The model under review builds one solid part; all positions refer to its coordinate system, in mm. A direction names the side the tool comes from. Give positions to 0.01 mm unless a question says otherwise; leave off trailing zeros. Write each loop counter-clockwise with the first axis right and the second up, starting at its lowest first coordinate (ties: lowest second). Pieces come first, ordered by that corner, then holes. Notation, with made-up numbers: M 68,-38 L 98,-38 A22 cw 98,-18 Z; hole C 12,79 d2. An arc over 180 degrees is marked long. Write item = value, one per line. Start each with the question number.
```python
from build123d import *

# Parameters (mm, degrees)
SKETCH1_W           = 10
SKETCH1_H           = 50
BOSS_EXTRUDE1_DEPTH = 2
SKETCH2_R           = 3
CUT_EXTRUDE1_DEPTH  = 2
SKETCH3_R           = 3
BOSS_EXTRUDE2_DEPTH = 20


with BuildPart() as part:
    # Sketch1 → Boss-Extrude1 (new body)
    with BuildSketch(Plane(origin=(0, 0, 0), x_dir=(0, 0, -1), z_dir=(1, 0, 0))):
        Rectangle(SKETCH1_W, SKETCH1_H)
    extrude(amount=BOSS_EXTRUDE1_DEPTH)

    # Sketch2 → Cut-Extrude1 (cut)
    with BuildSketch(Plane(origin=(2, 0, 0), x_dir=(0, 0, -1), z_dir=(1, 0, 0))):
        with Locations((0, 20)):
            Circle(SKETCH2_R)
    extrude(amount=-CUT_EXTRUDE1_DEPTH, mode=Mode.SUBTRACT)

    # Sketch3 → Boss-Extrude2 (add)
    with BuildSketch(Plane(origin=(2, 0, 0), x_dir=(0, 0, -1), z_dir=(1, 0, 0))):
        with Locations((0, -20)):
            Circle(SKETCH3_R)
    extrude(amount=BOSS_EXTRUDE2_DEPTH)


solid = part.part
```
Item 1: For faces 1 (the cylindrical face through (11.86, -22.93, 0.65)), 2 (the flat face through (22, -20, 0)), list the 3-axis set-ups (+Z, -Z, +X, -X, +Y, -Y) from which the entire face can be reached by the end or side of a thin tool; tool diameter is ignored.
Item 2: Clearance check with flat-ended pins moving along their axes: P1, Ø3.5, axis at y = 20, z = 0, coming from the -X side; P2, Ø5, axis at x = 10.5, z = -3.5, coming from the -Y side; P3, Ø6, axis at x = 14, y = -19.5, coming from the +Z side. State where each tip first meets the part, or that it passes through.
Item 3: We need section B-B, the plane y = 20. Write out the cut boundary in (x, z), and give its area (3 significant figures).
Item 4: We need section D-D, the plane x = 10.5. Write out the cut boundary in (y, z).
Item 5: We need section A-A, the plane z = 0. Write out the cut boundary in (x, y), and give its area (3 significant figures).
Item 6: To check wall thickness, follow probe 1 along Y at (x, z) = (1.3, 0); probe 2 along X at (y, z) = (-9, -0.25); probe 3 along Y at (x, z) = (19, -1.5). State the ranges of each line that lie inside material, in increasing order. Write a range as [from, to].
Item 7: We need section C-C, the plane y = -20. Write out the cut boundary in (x, z).
Worked out:
q1.face_1 = +X
q1.face_2 = +Z, -Z, +X, +Y, -Y
q2.P1 = through
q2.P2 = -22.83
q2.P3 = 3
q3.outline = M 0,-5 L 2,-5 L 2,-3 L 0,-3 Z; M 0,3 L 2,3 L 2,5 L 0,5 Z
q3.area = 8.00 mm²
q4.outline = C -20,0 d6
q5.outline = M 0,-25 L 2,-25 L 2,-23 L 22,-23 L 22,-17 L 2,-17 L 2,17 L 0,17 Z; M 0,23 L 2,23 L 2,25 L 0,25 Z
q5.area = 208 mm²
q6.probe_1 = [-25, 17], [23, 25]
q6.probe_2 = [0, 2]
q6.probe_3 = [-22.6, -17.4]
q7.outline = M 0,-5 L 2,-5 L 2,-3 L 22,-3 L 22,3 L 2,3 L 2,5 L 0,5 Z
